Can you work these out from the model? Positions are in its coordinate system, mm. Give positions to 0.01 mm unless a question says otherwise; leave off trailing zeros. Order: outer loops, then holes, each group sorted by start corner. A loop starts at its lowest first (then second) coordinate and runs counter-clockwise, first axis right, second up.
Item 1: I want a section at D-D, the plane x = -26. Write out the boundary of the cut face in (y, z).
Item 2: I want a section at C-C, the plane y = 35. Write out the boundary of the cut face in (x, z), then the cut area to 3 significant figures.
Item 3: I'm going to push flat-ended pins straight in: pin 1 Ø2.5 at (y, z) = (-29, 1.5) entering from -X; pin 2 Ø1.5 at (x, z) = (-64.5, 3.5) entering from -Y; pin 3 Ø5 at (x, y) = (0, 66.14) entering from +Z; pin 4 Ø2.5 at (x, z) = (69, 2.5) entering from -Y. Where does each tip first touch, or does it pass through?
Item 4: I want a section at B-B, the plane z = 3.2. Write out the boundary of the cut face in (x, y).
Item 5: I want a section at A-A, the plane x = 0. Write out the boundary of the cut face in (y, z).
Item 6: If I drill on line 1 along Y through (x, z) = (0, 1.65); line 2 along Y through (x, z) = (-0.5, 2.6); line 3 along X through (y, z) = (-50.5, 3), over which ranges is the centre line in solid material (lowest first)?
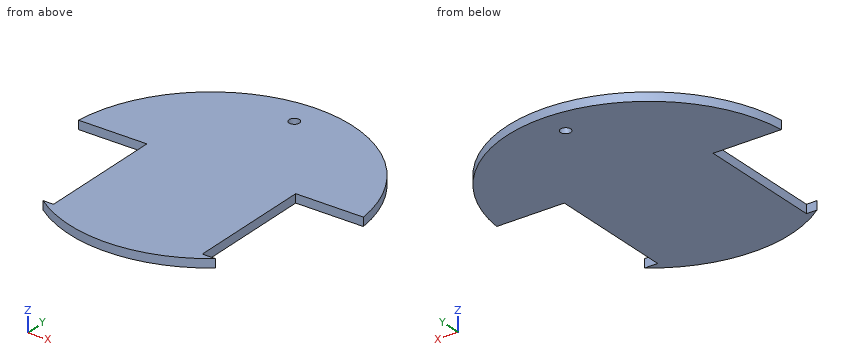
```python
from build123d import *

# Parameters (mm, degrees)
SKETCH_R     = 82.5
PAD_DEPTH    = 5
SKETCH001_W  = 40
SKETCH001_H  = 74
POCKET_DEPTH = 5
SKETCH002_R  = 3
HOLE_DEPTH   = 25


with BuildPart() as part:
    # Sketch → Pad (new body)
    with BuildSketch(Plane.XY):
        Circle(SKETCH_R)
    extrude(amount=PAD_DEPTH)

    # Sketch001 (on Face3 of Pad) → Pocket (cut)
    with BuildSketch(Plane.XY.offset(5)):
        with Locations((-62.53936, -29.626459)):
            Rectangle(SKETCH001_W, SKETCH001_H)
        with Locations((62.773894, -28.234338)):
            Rectangle(SKETCH001_W, SKETCH001_H)
    extrude(amount=-POCKET_DEPTH, mode=Mode.SUBTRACT)

    # Sketch002 (on Face4 of Pocket) → Hole (cut)
    with BuildSketch(Plane.XY.offset(5)):
        with Locations((0, 66.137764)):
            Circle(SKETCH002_R)
    extrude(amount=-HOLE_DEPTH, mode=Mode.SUBTRACT)


solid = part.part
```
Results list:
1. outline: (-78.3, 0) - (78.3, 0) - (78.3, 5) - (-78.3, 5) - close
2. outline: (-74.71, 0) - (74.71, 0) - (74.71, 5) - (-74.71, 5) - close
2. area: 747 mm2
3. pin 1: stops at x = -42.54
3. pin 2: stops at y = 7.37
3. pin 3: passes through
3. pin 4: stops at y = 8.77
4. outline: (-82.17, 7.37) - (-42.54, 7.37) - (-42.54, -66.63) - (-48.65, -66.63) arc R82.5 ccw to (50.5, -65.23) - (42.77, -65.23) - (42.77, 8.77) - (82.03, 8.77) arc R82.5 ccw to start; hole circle Ø6 at (0, 66.14)
5. outline: (-82.5, 0) - (63.14, 0) - (63.14, 5) - (-82.5, 5) - close; (69.14, 0) - (82.5, 0) - (82.5, 5) - (69.14, 5) - close
6. line 1: y = -82.5 to 63.14, 69.14 to 82.5
6. line 2: y = -82.5 to 63.18, 69.1 to 82.5
6. line 3: x = -42.54 to 42.77
